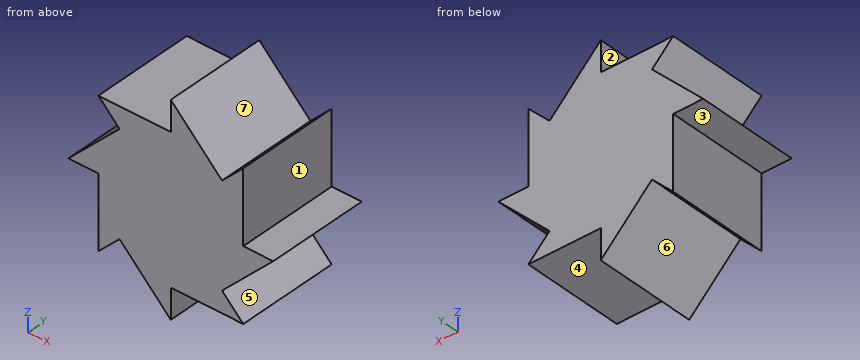
```python
from build123d import *

# Parameters (mm, degrees)
SKETCH1_R           = 5
BOSS_EXTRUDE1_DEPTH = 5
CUT_EXTRUDE1_DEPTH  = 9.660254038
CIRPATTERN1_COUNT   = 8


with BuildPart() as part:
    # Sketch1 → Boss-Extrude1 (new body)
    with BuildSketch(Plane(origin=(0, 0, 0), x_dir=(1, 0, 0), z_dir=(0, 1, 0))):
        with Locations(Location((0, 0, 0), (0, 0, 270))):
            Circle(SKETCH1_R)
    extrude(amount=BOSS_EXTRUDE1_DEPTH)

    # Sketch2 → Cut-Extrude1 (cut, through all)
    with BuildSketch(Plane(origin=(0, 5, 0), x_dir=(1, 0, 0), z_dir=(0, 1, 0))):
        with BuildLine():
            Line((0, 5), (0, 3.535533906))
            Line((0, 3.535533906), (3.535533906, 3.535533906))
            ThreePointArc((3.535533906, 3.535533906), (1.913417162, 4.619397663), (0, 5))
        make_face()
    cut_extrude1 = extrude(amount=-CUT_EXTRUDE1_DEPTH, mode=Mode.SUBTRACT)

    # CirPattern1: Cut-Extrude1 ×8 about axis
    cirpattern1_axis = Axis((0, 0, 0), (0, 1, 0))
    for i in range(1, CIRPATTERN1_COUNT):
        add(cut_extrude1.rotate(cirpattern1_axis, i * 360 / CIRPATTERN1_COUNT), mode=Mode.SUBTRACT)


solid = part.part
```
CAD build for the part. Positions are in the model's coordinates, mm. Face numbers are marked on the shaded views. A direction names the side the tool comes from. Coordinates: 2 decimals unless noted, no trailing zeros. Order: outer loops, then holes, each group sorted by start corner. A loop starts at its lowest first (then second) coordinate and runs counter-clockwise, first axis right, second up. Notation, with made-up numbers: (79, 66) -> (107, 66) arc R6 ccw to (107, 77) -> close; hole circle Ø6 at (17.5, 9). An arc over 180 degrees is marked (long way). Use one line per item in the form item = value. Start each with the question number.
1) Pull direction Z, two halves, no side cores. Call the marked faces 5, 6 and 7: +Z half, -Z half, draft (parallel to the pull), parting line (faces both ways), or undercut.
2) Band-saw the part on B-B on y = 2.7. Give the cut face in (x, z).
3) Band-saw the part on C-C on x = -4.25. Give the cut face in (y, z).
4) Drill centre lines: L1, parallel to Z at x = 0.5, y = 1; L2, parallel to Z at x = 2.25, y = 2.7; L3, parallel to X at y = 2.8, z = 1.25. Where is each one in solid material? Low to high. Write a range as [from, to].
5) Tool access for the marked faces 1, 2, 3 and 4: list every direction of +Z, -Z, +X, -X, +Y, -Y with a clear straight run to the whole face (end or side of a thin tool).
6) Band-saw the part on D-D on z = 1.5. Give the cut face in (x, y), then the cut area to 3 significant figures.
7) Band-saw the part on A-A on z = -3. Give the cut face in (x, y).
8) Drop flat-ended pins along their axis: pin 1 (1.6 mm diameter, centred on x = 4, y = 3.5, fed in from +Z); pin 2 (1.6 mm diameter, centred on y = 3, z = -4.5, fed in from +X); pin 3 (2 mm diameter, centred on y = 1, z = 3.5, fed in from -X). Give the stop position or say it passes through.
Entries:
q1.face_5 = undercut
q1.face_6 = -Z half
q1.face_7 = +Z half
q2.outline = (-5, 0) -> (-3.54, 0) -> (-3.54, -3.54) -> (-2.5, -2.5) -> (0, -5) -> (0, -3.54) -> (3.54, -3.54) -> (2.5, -2.5) -> (5, 0) -> (3.54, 0) -> (3.54, 3.54) -> (2.5, 2.5) -> (0, 5) -> (0, 3.54) -> (-3.54, 3.54) -> (-2.5, 2.5) -> close
q3.outline = (0, 0) -> (5, 0) -> (5, 0.75) -> (0, 0.75) -> close
q4.L1 = [-3.54, 4.5]
q4.L2 = [-3.54, 2.75]
q4.L3 = [-3.75, 3.54]
q5.face_1 = +Z, +X, +Y, -Y
q5.face_2 = +Z, -X, +Y, -Y
q5.face_3 = -Z, -X, +Y, -Y
q5.face_4 = -Z, +X, +Y, -Y
q6.outline = (-3.5, 0) -> (3.54, 0) -> (3.54, 5) -> (-3.5, 5) -> close
q6.area = 35.2 mm2
q7.outline = (-3.54, 0) -> (-3, 0) -> (-3, 5) -> (-3.54, 5) -> close; (-2, 0) -> (3, 0) -> (3, 5) -> (-2, 5) -> close
q8.pin_1 = 3.54
q8.pin_2 = 0
q8.pin_3 = -3.54
